```python
from build123d import *

# Parameters (mm, degrees)
BOSS_EXTRUDE1_DEPTH             = 2000
SKETCH2_W                       = 115000
SKETCH2_H                       = 70000
CUT_EXTRUDE1_DEPTH              = 2001
SKETCH3_W                       = 2250
SKETCH3_H                       = 50000
BOSS_EXTRUDE2_DEPTH             = 4000
SKETCH4_W                       = 90000
SKETCH4_H                       = 2250
BOSS_EXTRUDE3_DEPTH             = 4000
SKETCH5_W                       = 90000
SKETCH5_H                       = 2250
BOSS_EXTRUDE4_DEPTH             = 4000
SKETCH6_W                       = 2250
SKETCH6_H                       = 50000
BOSS_EXTRUDE5_DEPTH             = 4000
SCALE4_SCALE                    = 0.001
SKETCH17_W                      = 4
SKETCH17_H                      = 50
BOSS_EXTRUDE7_DEPTH             = 4
F_40_0_098_DIAMETER_HOLE1_D     = 2.50000008
F_40_0_098_DIAMETER_HOLE1_DEPTH = 3
F_40_0_098_DIAMETER_HOLE1_TIP   = 0.751075798
SKETCH21_W                      = 90
SKETCH21_H                      = 4
BOSS_EXTRUDE8_DEPTH             = 4
SKETCH22_W                      = 4
SKETCH22_H                      = 50
BOSS_EXTRUDE9_DEPTH             = 4
SKETCH23_W                      = 90
SKETCH23_H                      = 4
BOSS_EXTRUDE10_DEPTH            = 4
M2_5_CLEARANCE_HOLE3_D          = 2.9
M2_5_CLEARANCE_HOLE3_DEPTH      = 3
M2_5_CLEARANCE_HOLE3_TIP        = 0.871247898
M2_5_CLEARANCE_HOLE4_D          = 2.9
M2_5_CLEARANCE_HOLE4_DEPTH      = 3
M2_5_CLEARANCE_HOLE4_TIP        = 0.871247898
M2_5_CLEARANCE_HOLE5_D          = 2.9
M2_5_CLEARANCE_HOLE5_DEPTH      = 3
M2_5_CLEARANCE_HOLE5_TIP        = 0.871247898


with BuildPart() as part:
    # Sketch1 → Boss-Extrude1 (new body)
    with BuildSketch(Plane(origin=(0, 0, 66500), x_dir=(-1, 0, 0), z_dir=(0, 0, -1))):
        Polygon((41099.998474121, 59322.700500488), (37318.000793457, 61033.9012146), (33433.799743652, 62577.899932861), (29457.799911499, 63950.298309326), (25401.19934082, 65147.399902344), (21274.900436401, 66165.901184082), (17090.299606323, 67003.09753418), (12858.90007019, 67656.600952148), (8592.240333557, 68124.702453613), (4302.020072937, 68406.097412109), (0, 68500), (-4302.020072937, 68406.097412109), (-8592.240333557, 68124.702453613), (-12858.90007019, 67656.600952148), (-17090.299606323, 67003.09753418), (-21274.900436401, 66165.901184082), (-25401.19934082, 65147.399902344), (-29457.799911499, 63950.298309326), (-33433.799743652, 62577.899932861), (-37318.000793457, 61033.9012146), (-41099.998474121, 59322.700500488), (-44769.298553467, 57448.89831543), (-48315.898895264, 55417.701721191), (-51730.098724365, 53234.50088501), (-55002.498626709, 50905.39932251), (-58124.198913574, 48436.798095703), (-61086.498260498, 45835.399627686), (-63881.401062012, 43108.3984375), (-66501.197814941, 40263.301849365), (-68938.697814941, 37307.800292969), (-71187.301635742, 34250), (-73240.699768066, 31098.300933838), (-75093.399047852, 27861.499786377), (-76740.303039551, 24548.2006073), (-78176.803588867, 21167.699813843), (-79399.101257324, 17729.099273682), (-80403.701782227, 14241.99962616), (-81188.003540039, 10715.800285339), (-81749.702453613, 7160.200119019), (-82087.303161621, 3585.010051727), (-82199.996948242, 0), (-82087.303161621, -3585.010051727), (-81749.702453613, -7160.200119019), (-81188.003540039, -10715.800285339), (-80403.701782227, -14241.99962616), (-79399.101257324, -17729.099273682), (-78176.803588867, -21167.699813843), (-76740.303039551, -24548.2006073), (-75093.399047852, -27861.499786377), (-73240.699768066, -31098.300933838), (-71187.301635742, -34250), (-68938.697814941, -37307.800292969), (-66501.197814941, -40263.301849365), (-63881.401062012, -43108.3984375), (-61086.498260498, -45835.399627686), (-58124.198913574, -48436.798095703), (-55002.498626709, -50905.39932251), (-51730.098724365, -53234.50088501), (-48315.898895264, -55417.701721191), (-44769.298553467, -57448.89831543), (-41099.998474121, -59322.700500488), (-37318.000793457, -61033.9012146), (-33433.799743652, -62577.899932861), (-29457.799911499, -63950.298309326), (-25401.19934082, -65147.399902344), (-21274.900436401, -66165.901184082), (-17090.299606323, -67003.09753418), (-12858.90007019, -67656.600952148), (-8592.240333557, -68124.702453613), (-4302.020072937, -68406.097412109), (0, -68500), (4302.020072937, -68406.097412109), (8592.240333557, -68124.702453613), (12858.90007019, -67656.600952148), (17090.299606323, -67003.09753418), (21274.900436401, -66165.901184082), (25401.19934082, -65147.399902344), (29457.799911499, -63950.298309326), (33433.799743652, -62577.899932861), (37318.000793457, -61033.9012146), (41099.998474121, -59322.700500488), (44769.298553467, -57448.89831543), (48315.898895264, -55417.701721191), (51730.098724365, -53234.50088501), (55002.498626709, -50905.39932251), (58124.198913574, -48436.798095703), (61086.498260498, -45835.399627686), (63881.401062012, -43108.3984375), (66501.197814941, -40263.301849365), (68938.697814941, -37307.800292969), (71187.301635742, -34250), (73240.699768066, -31098.300933838), (75093.399047852, -27861.499786377), (76740.303039551, -24548.2006073), (78176.803588867, -21167.699813843), (79399.101257324, -17729.099273682), (80403.701782227, -14241.99962616), (81188.003540039, -10715.800285339), (81749.702453613, -7160.200119019), (82087.303161621, -3585.010051727), (82199.996948242, 0), (82087.303161621, 3585.010051727), (81749.702453613, 7160.200119019), (81188.003540039, 10715.800285339), (80403.701782227, 14241.99962616), (79399.101257324, 17729.099273682), (78176.803588867, 21167.699813843), (76740.303039551, 24548.2006073), (75093.399047852, 27861.499786377), (73240.699768066, 31098.300933838), (71187.301635742, 34250), (68938.697814941, 37307.800292969), (66501.197814941, 40263.301849365), (63881.401062012, 43108.3984375), (61086.498260498, 45835.399627686), (58124.198913574, 48436.798095703), (55002.498626709, 50905.39932251), (51730.098724365, 53234.50088501), (48315.898895264, 55417.701721191), (44769.298553467, 57448.89831543), align=None)
    extrude(amount=-BOSS_EXTRUDE1_DEPTH)

    # Sketch2 → Cut-Extrude1 (cut, through all)
    with BuildSketch(Plane.XY.offset(68500)):
        Rectangle(SKETCH2_W, SKETCH2_H)
    extrude(amount=-CUT_EXTRUDE1_DEPTH, mode=Mode.SUBTRACT)

    # Sketch3 → Boss-Extrude2 (add)
    with BuildSketch(Plane(origin=(0, 0, 66500), x_dir=(-1, 0, 0), z_dir=(0, 0, -1))):
        with Locations((62375, 0)):
            Rectangle(SKETCH3_W, SKETCH3_H)
    extrude(amount=BOSS_EXTRUDE2_DEPTH)

    # Sketch4 → Boss-Extrude3 (add)
    with BuildSketch(Plane(origin=(0, 0, 66500), x_dir=(-1, 0, 0), z_dir=(0, 0, -1))):
        with Locations((0, 39875)):
            Rectangle(SKETCH4_W, SKETCH4_H)
    extrude(amount=BOSS_EXTRUDE3_DEPTH)

    # Sketch5 → Boss-Extrude4 (add)
    with BuildSketch(Plane(origin=(0, 0, 66500), x_dir=(-1, 0, 0), z_dir=(0, 0, -1))):
        with Locations((0, -39875)):
            Rectangle(SKETCH5_W, SKETCH5_H)
    extrude(amount=BOSS_EXTRUDE4_DEPTH)

    # Sketch6 → Boss-Extrude5 (add)
    with BuildSketch(Plane(origin=(0, 0, 66500), x_dir=(-1, 0, 0), z_dir=(0, 0, -1))):
        with Locations((-62375, 0)):
            Rectangle(SKETCH6_W, SKETCH6_H)
    extrude(amount=BOSS_EXTRUDE5_DEPTH)


with BuildPart() as part_1:
    # Scale4: scaled about (0, 0, 67152.933263132)
    add(part.part.scale(SCALE4_SCALE).moved(Location((0, 0, 67085.780329869))))

    # Sketch17 → Boss-Extrude7 (add)
    with BuildSketch(Plane(origin=(0, 0, 67152.280329869), x_dir=(-1, 0, 0), z_dir=(0, 0, -1))):
        with Locations((-63.25, 0)):
            Rectangle(SKETCH17_W, SKETCH17_H)
    extrude(amount=BOSS_EXTRUDE7_DEPTH)

    # #40 (0.098) Diameter Hole1
    with Locations(Plane(origin=(0, 0, 67148.280329869), x_dir=(-1, 0, 0), z_dir=(0, 0, -1))):
        with Locations((-63.25, 0)):
            Hole(F_40_0_098_DIAMETER_HOLE1_D / 2, depth=F_40_0_098_DIAMETER_HOLE1_DEPTH)
            with Locations((0, 0, -(F_40_0_098_DIAMETER_HOLE1_DEPTH + F_40_0_098_DIAMETER_HOLE1_TIP / 2))):  # 118° drill point
                Cone(0, F_40_0_098_DIAMETER_HOLE1_D / 2, F_40_0_098_DIAMETER_HOLE1_TIP, mode=Mode.SUBTRACT)

    # Sketch21 → Boss-Extrude8 (add)
    with BuildSketch(Plane(origin=(0, 0, 67152.280329869), x_dir=(-1, 0, 0), z_dir=(0, 0, -1))):
        with Locations((0, 40.75)):
            Rectangle(SKETCH21_W, SKETCH21_H)
    extrude(amount=BOSS_EXTRUDE8_DEPTH)

    # Sketch22 → Boss-Extrude9 (add)
    with BuildSketch(Plane(origin=(0, 0, 67152.280329869), x_dir=(-1, 0, 0), z_dir=(0, 0, -1))):
        with Locations((63.25, 0)):
            Rectangle(SKETCH22_W, SKETCH22_H)
    extrude(amount=BOSS_EXTRUDE9_DEPTH)

    # Sketch23 → Boss-Extrude10 (add)
    with BuildSketch(Plane(origin=(0, 0, 67152.280329869), x_dir=(-1, 0, 0), z_dir=(0, 0, -1))):
        with Locations((0, -40.75)):
            Rectangle(SKETCH23_W, SKETCH23_H)
    extrude(amount=BOSS_EXTRUDE10_DEPTH)

    # M2.5 Clearance Hole3
    with Locations(Plane(origin=(0, 0, 67148.280329869), x_dir=(-1, 0, 0), z_dir=(0, 0, -1))):
        with Locations((0, -40.75)):
            Hole(M2_5_CLEARANCE_HOLE3_D / 2, depth=M2_5_CLEARANCE_HOLE3_DEPTH)
            with Locations((0, 0, -(M2_5_CLEARANCE_HOLE3_DEPTH + M2_5_CLEARANCE_HOLE3_TIP / 2))):  # 118° drill point
                Cone(0, M2_5_CLEARANCE_HOLE3_D / 2, M2_5_CLEARANCE_HOLE3_TIP, mode=Mode.SUBTRACT)

    # M2.5 Clearance Hole4
    with Locations(Plane(origin=(0, 0, 67148.280329869), x_dir=(-1, 0, 0), z_dir=(0, 0, -1))):
        with Locations((0, 40.75)):
            Hole(M2_5_CLEARANCE_HOLE4_D / 2, depth=M2_5_CLEARANCE_HOLE4_DEPTH)
            with Locations((0, 0, -(M2_5_CLEARANCE_HOLE4_DEPTH + M2_5_CLEARANCE_HOLE4_TIP / 2))):  # 118° drill point
                Cone(0, M2_5_CLEARANCE_HOLE4_D / 2, M2_5_CLEARANCE_HOLE4_TIP, mode=Mode.SUBTRACT)

    # M2.5 Clearance Hole5
    with Locations(Plane(origin=(0, 0, 67148.280329869), x_dir=(-1, 0, 0), z_dir=(0, 0, -1))):
        with Locations((63.25, 0)):
            Hole(M2_5_CLEARANCE_HOLE5_D / 2, depth=M2_5_CLEARANCE_HOLE5_DEPTH)
            with Locations((0, 0, -(M2_5_CLEARANCE_HOLE5_DEPTH + M2_5_CLEARANCE_HOLE5_TIP / 2))):  # 118° drill point
                Cone(0, M2_5_CLEARANCE_HOLE5_D / 2, M2_5_CLEARANCE_HOLE5_TIP, mode=Mode.SUBTRACT)


solid = part_1.part
```
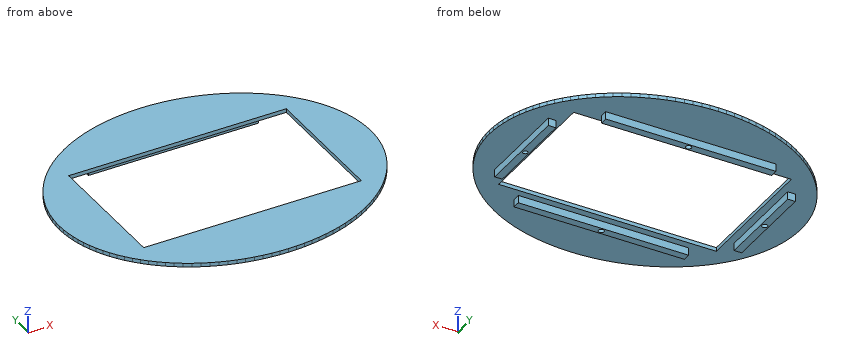
Work out the finished part from the listing and answer in its coordinate system (mm). Give positions to 0.01 mm unless a question says otherwise; leave off trailing zeros. Loops run counter-clockwise (first coordinate to the right, second up) from the corner with the lowest first, then second, coordinate; pieces in that order, holes last. Notation, with made-up numbers: (-15, -6) - (14, -6) arc R13 cw to (14, 16) - close; hole circle Ø5 at (-12, 78.25). An arc over 180 degrees is marked (long way). Use CSV: the item, a comma, the result in double quotes. Start each with the question number.
(1) Find section A-A, the plane z = 67149.75. Determine the outline of the cut face in (x, y), plus the area to 3 significant figures.
(2) Find section B-B, the plane y = 12.5. Determine the outline of the cut face in (x, z), plus the area to 3 significant figures.
(3) Find the intervals of material crossed by L1, parallel to X at y = 0, z = 67149.6; L2, parallel to Y at x = 0, z = 67149.45; L3, parallel to Y at x = -63.25, z = 67148.9, in increasing order.
(4) Each of these flat-tipped pins is pushed along its axis until it touches: pin 1 (1.2 mm diameter, centred on x = -6, z = 67150.5, fed in from -Y); pin 2 (2 mm diameter, centred on x = 4.5, z = 67150, fed in from +Y); pin 3 (8 mm diameter, centred on x = -36, y = 50, fed in from -Z). Where does it stop, or does it pass through?
Results found:
1,outline,"(-65.25, -25) - (-61.25, -25) - (-61.25, 25) - (-65.25, 25) - close; (-45, -42.75) - (45, -42.75) - (45, -38.75) - (-45, -38.75) - close; (-45, 38.75) - (45, 38.75) - (45, 42.75) - (-45, 42.75) - close; (61.25, -25) - (65.25, -25) - (65.25, 25) - (61.25, 25) - close; hole circle Ø2.9 at (-63.25, 0); hole circle Ø2.9 at (0, -40.75); hole circle Ø2.9 at (0, 40.75); hole circle Ø2.5 at (63.25, 0)"
1,area,"1,100 mm^2"
2,outline,"(-80.79, 67152.28) - (-65.25, 67152.28) - (-65.25, 67148.28) - (-61.25, 67148.28) - (-61.25, 67152.28) - (-57.5, 67152.28) - (-57.5, 67154.28) - (-80.79, 67154.28) - close; (57.5, 67152.28) - (61.25, 67152.28) - (61.25, 67148.28) - (65.25, 67148.28) - (65.25, 67152.28) - (80.79, 67152.28) - (80.79, 67154.28) - (57.5, 67154.28) - close"
2,area,"125 mm^2"
3,L1,"-65.25 to -64.7, -61.8 to -61.25, 61.25 to 62, 64.5 to 65.25"
3,L2,"-42.75 to -42.2, -39.3 to -38.75, 38.75 to 39.3, 42.2 to 42.75"
3,L3,"-25 to -1.45, 1.45 to 25"
4,pin 1,"y = -42.75"
4,pin 2,"y = 42.75"
4,pin 3,"z = 67152.28"
